from build123d import *

# Parameters (mm, degrees)
F0_R     = 1.5875
F1_DEPTH = 25.4


with BuildPart() as f1:
    # F0 (on Front) → F1 (new body)
    with BuildSketch(Plane.XZ):
        with BuildLine():
            ThreePointArc((9.525, 50.8), (6.7351920908, 44.0648079092), (0, 41.275))
            Line((0, 41.275), (0, 15.875))
            ThreePointArc((0, 15.875), (10.500263397, 11.9063047833), (15.7504675666, 1.9845393503))
            Line((15.7504675666, 1.9845393503), (9.4622685099, 51.8913751176))
            ThreePointArc((9.4622685099, 51.8913751176), (9.5093041953, 51.3465882562), (9.525, 50.8))
        make_face()
        with BuildLine():
            Line((0, 15.875), (0, 41.275))
            ThreePointArc((0, 41.275), (-7.0608217366, 44.4070021583), (-9.4781770336, 51.7432842197))
            Line((-9.4781770336, 51.7432842197), (-15.7503596183, 1.9853959035))
            ThreePointArc((-15.7503596183, 1.9853959035), (-10.4999396434, 11.9065902963), (0, 15.875))
        make_face()
        with Locations((-4.9275723286, 36.5252)):
            Circle(F0_R, mode=Mode.SUBTRACT)
        with BuildLine():
            ThreePointArc((15.7504675666, 1.9845393503), (10.500263397, 11.9063047833), (0, 15.875))
            Line((0, 15.875), (0, 3.5818445827))
            ThreePointArc((0, 3.5818445827), (2.5327465936, 2.5327465936), (3.5818445827, 0))
            ThreePointArc((3.5818445827, 0), (2.5327465936, -2.5327465936), (0, -3.5818445827))
            Line((0, -3.5818445827), (0, -15.875))
            ThreePointArc((0, -15.875), (11.2253201513, -11.2253201513), (15.875, 0))
            ThreePointArc((15.875, 0), (15.8438363034, 0.9942213988), (15.7504675666, 1.9845393503))
        make_face()
        with BuildLine():
            Line((0, 3.5818445827), (0, 15.875))
            ThreePointArc((0, 15.875), (-10.4999396434, 11.9065902963), (-15.7503596183, 1.9853959035))
            ThreePointArc((-15.7503596183, 1.9853959035), (-11.9065902963, -10.4999396434), (0, -15.875))
            Line((0, -15.875), (0, -3.5818445827))
            ThreePointArc((0, -3.5818445827), (-3.5818445827, 0), (0, 3.5818445827))
        make_face()
        with BuildLine():
            ThreePointArc((0, -15.875), (-11.9065902963, -10.4999396434), (-15.7503596183, 1.9853959035))
            Line((-15.7503596183, 1.9853959035), (-16.0006267826, 0))
            Line((-16.0006267826, 0), (-9.5283009961, -64.4567694559))
            ThreePointArc((-9.5283009961, -64.4567694559), (-7.1016251441, -57.0757609029), (0, -53.923783228))
            Line((0, -53.923783228), (0, -15.875))
        make_face()
        with BuildLine():
            Line((16.0005170494, 0), (15.7504675666, 1.9845393503))
            ThreePointArc((15.7504675666, 1.9845393503), (15.8438363034, 0.9942213988), (15.875, 0))
            ThreePointArc((15.875, 0), (11.2253201513, -11.2253201513), (0, -15.875))
            Line((0, -15.875), (0, -53.923783228))
            ThreePointArc((0, -53.923783228), (6.7714078176, -56.7285921824), (9.576216772, -63.5))
            Line((9.576216772, -63.5), (36.5125, -63.5))
            ThreePointArc((36.5125, -63.5), (38.9413556042, -57.7852171371), (44.7414746571, -55.5678534573))
            Line((44.7414746571, -55.5678534573), (18.9771161719, -54.6211163395))
            ThreePointArc((18.9771161719, -54.6211163395), (13.2743662579, -51.8982857051), (11.3592341777, -45.876040911))
            Line((11.3592341777, -45.876040911), (16.0005170494, 0))
        make_face()
        with BuildLine():
            Line((36.5125, -63.5), (9.576216772, -63.5))
            ThreePointArc((9.576216772, -63.5), (7.0154951661, -70.0181864992), (0.7028263194, -73.050390716))
            Line((0.7028263194, -73.050390716), (44.7414746571, -71.4321465427))
            ThreePointArc((44.7414746571, -71.4321465427), (38.9413556042, -69.2147828629), (36.5125, -63.5))
        make_face()
        with BuildLine():
            ThreePointArc((-9.4781770336, 51.7432842197), (-7.0608217366, 44.4070021583), (0, 41.275))
            ThreePointArc((0, 41.275), (6.7351920908, 44.0648079092), (9.525, 50.8))
            ThreePointArc((9.525, 50.8), (9.5093041953, 51.3465882562), (9.4622685099, 51.8913751176))
            Line((9.4622685099, 51.8913751176), (9.4372495094, 52.089940579))
            ThreePointArc((9.4372495094, 52.089940579), (0.0749897766, 60.3247048003), (-9.4157689808, 52.2383739084))
            Line((-9.4157689808, 52.2383739084), (-9.4781770336, 51.7432842197))
        make_face()
        with BuildLine():
            ThreePointArc((3.2273454684, 50.8), (2.282077866, 48.517922134), (0, 47.5726545316))
            ThreePointArc((0, 47.5726545316), (-2.282077866, 53.082077866), (3.2273454684, 50.8))
        make_face(mode=Mode.SUBTRACT)
        with BuildLine():
            Line((0, -60.4259204753), (0, -53.923783228))
            ThreePointArc((0, -53.923783228), (-7.1016251441, -57.0757609029), (-9.5283009961, -64.4567694559))
            ThreePointArc((-9.5283009961, -64.4567694559), (-6.4242390971, -70.6016251441), (0, -73.076216772))
            Line((0, -73.076216772), (0.7028263194, -73.050390716))
            ThreePointArc((0.7028263194, -73.050390716), (7.0154951661, -70.0181864992), (9.576216772, -63.5))
            Line((9.576216772, -63.5), (3.0740795247, -63.5))
            ThreePointArc((3.0740795247, -63.5), (-2.1737024778, -65.6737024778), (0, -60.4259204753))
        make_face()
        with BuildLine():
            ThreePointArc((9.576216772, -63.5), (6.7714078176, -56.7285921824), (0, -53.923783228))
            Line((0, -53.923783228), (0, -60.4259204753))
            ThreePointArc((0, -60.4259204753), (2.1737024778, -61.3262975222), (3.0740795247, -63.5))
            Line((3.0740795247, -63.5), (9.576216772, -63.5))
        make_face()
        with BuildLine():
            ThreePointArc((52.3875, -63.5), (50.1647828629, -57.9913556042), (44.7414746571, -55.5678534573))
            ThreePointArc((44.7414746571, -55.5678534573), (38.9413556042, -57.7852171371), (36.5125, -63.5))
            ThreePointArc((36.5125, -63.5), (38.9413556042, -69.2147828629), (44.7414746571, -71.4321465427))
            ThreePointArc((44.7414746571, -71.4321465427), (50.1647828629, -69.0086443958), (52.3875, -63.5))
        make_face()
        with BuildLine():
            ThreePointArc((47.5920096932, -63.5), (44.45, -66.6420096932), (41.3079903068, -63.5))
            ThreePointArc((41.3079903068, -63.5), (44.45, -60.3579903068), (47.5920096932, -63.5))
        make_face(mode=Mode.SUBTRACT)
    extrude(amount=F1_DEPTH)


solid = f1.part
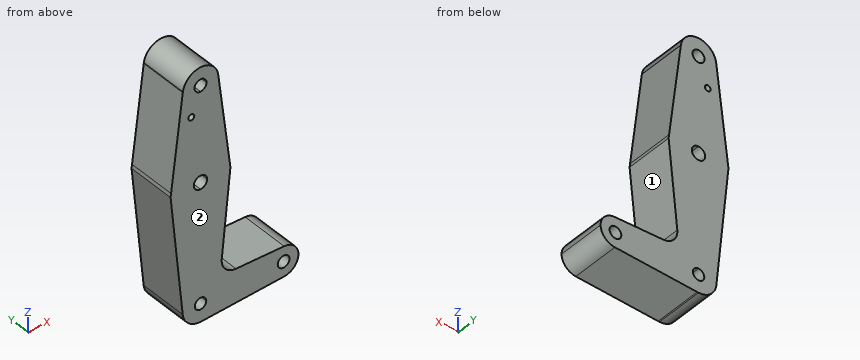
Check sheet for the modelled part. Datum: model origin and axes. Units: mm. Face numbers are marked on the shaded views. A direction names the side the tool comes from. Round coordinates to 2 decimals unless told otherwise and drop trailing zeros. Order: outer loops, then holes, each group sorted by start corner. A loop starts at its lowest first (then second) coordinate and runs counter-clockwise, first axis right, second up.
(1) Scan lines: probe 1 along Z at (x, y) = (44.45, -17.5); probe 2 along Z at (x, y) = (24.5, -18.75); probe 3 along X at (y, z) = (-13.75, -17.5). Record each from-to range of solid material in increasing order.
(2) Cross-section at B-B, the plane x = 28. Enter the section's corners in (y, z), and give its area (3 significant figures).
(3) Cross-section at C-C, the plane z = 12. Enter the section's corners in (x, y).
(4) Access from +Z, -Z, +X, -X, +Y, -Y to the whole of each face (thin tool, end or side, straight path). Record for the marked faces 1 and 2.
(5) Cross-section at A-A, the plane y = -15.5. State how many separate pieces and enclosed holes the cut face has, and give its area (3 significant figures).
(6) Go/stop test with flat-tipped pins: P1, Ø5, axis at x = 44.45, z = -63.5, coming from the +Y side; P2, Ø2, axis at x = 27, y = -12, coming from the +Z side; P3, Ø10, axis at y = -11, z = -36.5, coming from the +X side; P4, Ø3, axis at x = 2.5, z = 26, coming from the +Y side. Record where each tip stops, or that it passes through.
Check sheet entries:
1. probe 1: z = -71.44 to -66.64, -60.36 to -55.56
1. probe 2: z = -72.18 to -54.82
1. probe 3: x = -14.24 to 14.23
2. outline: (-25.4, -72.05) - (0, -72.05) - (0, -54.95) - (-25.4, -54.95) - close
2. area: 434 mm2
3. outline: (-14.49, -25.4) - (14.49, -25.4) - (14.49, 0) - (-14.49, 0) - close
4. face 1: +X, +Y, -Y
4. face 2: +Z, -Z, +X, -X, -Y
5. separate pieces: 1
5. enclosed holes: 5
5. area: 3,800 mm2
6. P1: passes through
6. P2: stops at z = -54.88
6. P3: stops at x = 12.81
6. P4: stops at y = 0
